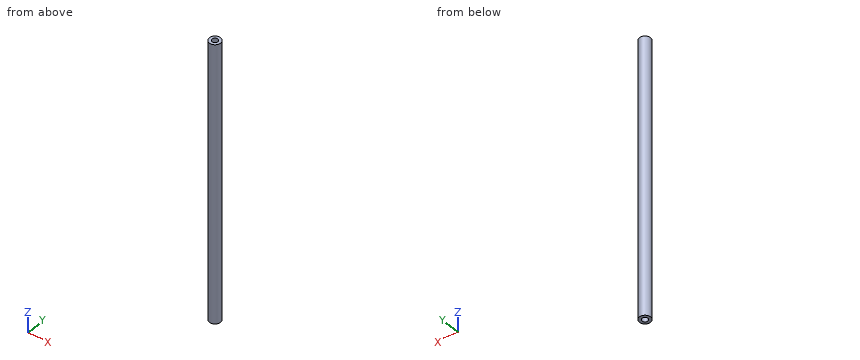
from build123d import *

# Parameters (mm, degrees)
F0_R     = 4
F1_DEPTH = 200
F3_D     = 4.2
F3_DEPTH = 14.4
F3_TIP   = 1.2618073
F5_D     = 4.2
F5_DEPTH = 14.4
F5_TIP   = 1.2618073


with BuildPart() as f1:
    # F0 (on Top) → F1 (new body)
    with BuildSketch(Plane.XY):
        Circle(F0_R)
    extrude(amount=F1_DEPTH)

    # F3
    with Locations(Plane.XY.offset(200)):
        with Locations((0, 0)):
            Hole(F3_D / 2, depth=F3_DEPTH)
            with Locations((0, 0, -(F3_DEPTH + F3_TIP / 2))):  # 118° drill point
                Cone(0, F3_D / 2, F3_TIP, mode=Mode.SUBTRACT)

    # F5
    with Locations(Plane(origin=(0, 0, 0), x_dir=(1, 0, 0), z_dir=(0, 0, -1))):
        with Locations((0, 0)):
            Hole(F5_D / 2, depth=F5_DEPTH)
            with Locations((0, 0, -(F5_DEPTH + F5_TIP / 2))):  # 118° drill point
                Cone(0, F5_D / 2, F5_TIP, mode=Mode.SUBTRACT)


solid = f1.part
Input: part model. Units: mm. Frame: model coordinates. Give positions to 0.01 mm unless a question says otherwise; leave off trailing zeros. Order: outer loops, then holes, each group sorted by start corner. A loop starts at its lowest first (then second) coordinate and runs counter-clockwise, first axis right, second up. Notation, with made-up numbers: (-37, 46.5) - (16, 46.5) arc R17 cw to (16, 78.5) - close; hole circle Ø2 at (57.25, -6). An arc over 180 degrees is marked (long way). Write each question's results on one line, items separated by ' | '.
Item 1: Contact query for flat-ended pins moving along their axis: pin 1 Ø1 at (y, z) = (3, 124.5) entering from -X; pin 2 Ø2.5 at (x, y) = (0, 0) entering from +Z; pin 3 Ø1 at (y, z) = (3, 163) entering from +X. Output: stop coordinate, or through.
A:
pin 1: stops at x = -3.12 | pin 2: stops at z = 185.09 | pin 3: stops at x = 3.12
Item 2: Material intervals for line 1 along Y through (x, z) = (0, 10.25); line 2 along Y through (x, z) = (-0.5, 50); line 3 along X through (y, z) = (0.5, 8.5), sorted ascending.
A:
line 1: y = -4 to -2.1, 2.1 to 4 | line 2: y = -3.97 to 3.97 | line 3: x = -3.97 to -2.04, 2.04 to 3.97
Item 3: Section A-A (z = 104.5). Return loops of the section in (x, y), and give its area (3 significant figures).
A:
outline: circle Ø8 at (0, 0) | area: 50.3 mm^2
